The listing builds one solid part. Answer for the finished solid, in the listing's coordinates (mm). A direction names the side the tool comes from. Round coordinates to 2 decimals unless told otherwise and drop trailing zeros. Write each loop counter-clockwise with the first axis right and the second up, starting at its lowest first coordinate (ties: lowest second). Pieces come first, ordered by that corner, then holes. Notation, with made-up numbers: (30.25, 23.25) - (79.25, 23.25) arc R21 cw to (79.25, 57.25) - close; hole circle Ø4 at (70, 77.5). An arc over 180 degrees is marked (long way). Return JSON: item names as keys, results as strings. Group by question number.
(1) Determine the mould class of faces 3 (the flat face through (60.325, -75, 62)), 4 (the flat face through (34, 0, 23)), 5 (the flat face through (-41.275, -75, 0)) for opening direction X: +X half, -X half, draft (parallel to the pull), parting line (faces both ways), or undercut.
(2) Each of these flat-tipped pins is pushed along its axis until it touches: pin 1 (4 mm diameter, centred on x = 12.5, y = -78, fed in from +Z); pin 2 (6 mm diameter, centred on x = 46.5, z = 23.5, fed in from +Y) (3 decimals); pin 3 (4 mm diameter, centred on x = 30.5, y = -81, fed in from +Z); pin 4 (1 mm diameter, centred on x = -24.5, y = -105.5, fed in from +Z). Where does it stop, or does it pass through?
(3) Find the intervals of material crossed by line 1 along Z through (x, y) = (96, -123) (3 decimals); line 2 along X through (y, z) = (-94, 3) (3 decimals); line 3 along X through (y, z) = (-76, 62) (3 decimals), in increasing order. Write a range as [from, to].
(4) Section A-A, the plane x = 76 is taken. Write down the section's boundary in (y, z) (3 decimals), then the cut area to 3 significant figures.
(5) Which of the six approach directions +Z, -Z, +X, -X, +Y, -Y give full straight-line access (tool end or side, diameter ignored) to faces 1 (the flat face through (84, -75, 34.925)), 2 (the flat face through (111.125, -75, 51))?
(6) Section B-B, the plane z = 61.5 is taken. Write down the section's boundary in (x, y) (3 decimals).
```python
from build123d import *

# Parameters (mm, degrees)
F1_DEPTH = 127
F2_DEPTH = 25.4


with BuildPart() as f1:
    # F0 (on Front) → F1 (new body)
    with BuildSketch(Plane.XZ):
        Polygon((-41.275, 9.525), (-41.275, -9.525), (41.275, -9.525), (41.275, 9.525), (22.225, 9.525), align=None)
        with BuildLine():
            add(Edge.make_bspline(
                [(-41.275, 9.525), (-8.6202568682, 9.525), (57.7562975598, 73.3467516444), (60.325, 56.3711255966)],
                knots=[0, 0, 0, 0, 106.6877251483, 106.6877251483, 106.6877251483, 106.6877251483], degree=3))
            Line((-41.275, 9.525), (22.225, 9.525))
            Line((22.225, 9.525), (22.225, 19.05))
            ThreePointArc((22.225, 19.05), (32.4542956671, 43.7457043329), (57.15, 53.975))
            Line((57.15, 53.975), (60.325, 53.975))
            Line((60.325, 53.975), (60.325, 56.3711255966))
        make_face()
        with BuildLine():
            Line((22.225, 9.525), (41.275, 9.525))
            Line((41.275, 9.525), (41.275, 19.05))
            ThreePointArc((41.275, 19.05), (45.9246798487, 30.2753201513), (57.15, 34.925))
            Line((57.15, 34.925), (60.325, 34.925))
            Line((60.325, 34.925), (60.325, 53.975))
            Line((60.325, 53.975), (57.15, 53.975))
            ThreePointArc((57.15, 53.975), (32.4542956671, 43.7457043329), (22.225, 19.05))
            Line((22.225, 19.05), (22.225, 9.525))
        make_face()
        with BuildLine():
            add(Edge.make_bspline(
                [(60.325, 56.3711255966), (60.4263696567, 55.7012101725), (60.4283676683, 54.9054643358), (60.325, 53.975)],
                knots=[106.6877251483, 106.6877251483, 106.6877251483, 106.6877251483, 110.8979823982, 110.8979823982, 110.8979823982, 110.8979823982], degree=3))
            Line((60.325, 56.3711255966), (60.325, 53.975))
        make_face()
        with BuildLine():
            Line((60.325, 66.675), (60.325, 56.3711255966))
            add(Edge.make_bspline(
                [(60.325, 56.3711255966), (60.4263696567, 55.7012101725), (60.4283676683, 54.9054643358), (60.325, 53.975)],
                knots=[106.6877251483, 106.6877251483, 106.6877251483, 106.6877251483, 110.8979823982, 110.8979823982, 110.8979823982, 110.8979823982], degree=3))
            Line((60.325, 53.975), (60.325, 34.925))
            Line((60.325, 34.925), (73.2388391052, 34.925))
            Line((73.2388391052, 34.925), (111.125, 34.925))
            Line((111.125, 34.925), (111.125, 66.675))
            Line((111.125, 66.675), (60.325, 66.675))
        make_face()
    extrude(amount=F1_DEPTH)

    # F2 (add): faces of the model
    f2_faces = [f1.faces().sort_by_distance(p)[0] for p in [
        (36.5781101492, -127, 26.7856673902),
        (36.5781101492, -127, 26.7856673902),
    ]]
    extrude(f2_faces, amount=F2_DEPTH)


solid = f1.part
```
Working result:
{
 "1": {"face 3": "undercut", "face 4": "draft", "face 5": "-X half"},
 "2": {"pin 1": "stops at z = 35.18", "pin 2": "passes through", "pin 3": "stops at z = 46.98", "pin 4": "stops at z = 13.6"},
 "3": {"line 1": "z = [34.925, 66.675]", "line 2": "x = [-41.275, 41.275]", "line 3": "x = [60.325, 111.125]"},
 "4": {"outline": "(-152.4, 34.925) - (0, 34.925) - (0, 66.675) - (-152.4, 66.675) - close", "area": "4,840 mm^2"},
 "5": {"face 1": "-Z, +X, +Y, -Y", "face 2": "+Z, -Z, +X, +Y, -Y"},
 "6": {"outline": "(60.325, -152.4) - (111.125, -152.4) - (111.125, 0) - (60.325, 0) - close"}
}
